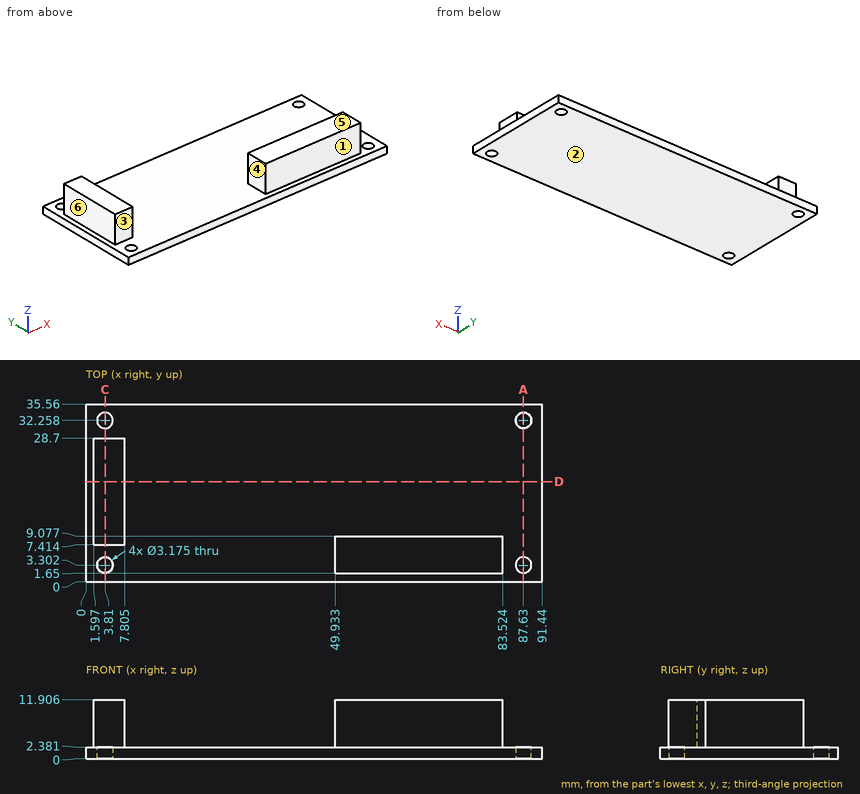
For this review, use the dimensioned drawing (mm, ordinates from the lowest corner) and the shaded views. A direction names the side the tool comes from. Coordinates: 2 decimals unless noted, no trailing zeros. Loops run counter-clockwise (first coordinate to the right, second up) from the corner with the lowest first, then second, coordinate; pieces in that order, holes last.
1. For the marked faces 1, 2 and 3, list the 3-axis set-ups (+Z, -Z, +X, -X, +Y, -Y) from which the entire face can be reached by the end or side of a thin tool; tool diameter is ignored.
2. Add section D-D, the plane y = 20. Give the boundary of the cut face in (x, z) (1 decimal), then the cut area to 3 significant figures.
3. Insertion check: P1, Ø1.5, axis at y = 16.5, z = 4, coming from the -X side; P2, Ø3, axis at x = 66.5, z = 5.5, coming from the +Y side; P3, Ø1, axis at x = 81.5, y = 32, coming from the +Z side. Each pin has a flat end and moves straight along its axis. Give the tip position at first contact, or say it passes through.
4. For line 1 (Y direction, x = 3.81, z = 1.1) (1 decimal); line 2 (X direction, y = 8.5, z = 5.5) (1 decimal); line 3 (Z direction, x = 11, y = 13.5), list the stretches that pass through material, from the lowest coordinate up.
5. Add section A-A, the plane x = 87.63. Give the boundary of the cut face in (y, z) (1 decimal).
6. Add section C-C, the plane x = 3.81. Give the boundary of the cut face in (y, z) (1 decimal), then the cut area to 3 significant figures.
7. Mouldability with a two-part tool opening along X and no side actions: class the marked faces 4, 5 and 6 as +X half, -X half, draft (parallel to the pull), parting line (faces both ways), or undercut.
Result:
1. face 1: +Z, +X, -X, -Y
1. face 2: -Z, +X, -X, +Y, -Y
1. face 3: +Z, -X, -Y
2. outline: (0, 0) - (91.4, 0) - (91.4, 2.4) - (7.8, 2.4) - (7.8, 11.9) - (1.6, 11.9) - (1.6, 2.4) - (0, 2.4) - close
2. area: 277 mm2
3. P1: stops at x = 1.6
3. P2: stops at y = 9.08
3. P3: stops at z = 2.38
4. line 1: y = 0 to 1.7, 4.9 to 30.7, 33.8 to 35.6
4. line 2: x = 1.6 to 7.8, 49.9 to 83.5
4. line 3: z = 0 to 2.38
5. outline: (0, 0) - (1.7, 0) - (1.7, 2.4) - (0, 2.4) - close; (4.9, 0) - (30.7, 0) - (30.7, 2.4) - (4.9, 2.4) - close; (33.8, 0) - (35.6, 0) - (35.6, 2.4) - (33.8, 2.4) - close
6. outline: (0, 0) - (1.7, 0) - (1.7, 2.4) - (0, 2.4) - close; (4.9, 0) - (30.7, 0) - (30.7, 2.4) - (28.7, 2.4) - (28.7, 11.9) - (7.4, 11.9) - (7.4, 2.4) - (4.9, 2.4) - close; (33.8, 0) - (35.6, 0) - (35.6, 2.4) - (33.8, 2.4) - close
6. area: 272 mm2
7. face 4: undercut
7. face 5: draft
7. face 6: -X half
